Could you check a few things on this model? Use its own coordinates, in mm. Coordinates: 2 decimals unless noted, no trailing zeros. Order: outer loops, then holes, each group sorted by start corner. A loop starts at its lowest first (then second) coordinate and runs counter-clockwise, first axis right, second up. Notation, with made-up numbers: (66, -14.5) - (86, -14.5) arc R17 cw to (86, 2.5) - close; hole circle Ø6 at (14, 63.5). An arc over 180 degrees is marked (long way). Answer as a JSON object with one key per item and string values. Group by question number.
(1) Imagine slicing it at B-B, the plane y = 26.5. Write out the boundary of the cut face in (x, z).
(2) Will these pins go through, and if not, where does the flat tip stop? P1, Ø1.5, axis at x = 1.5, y = -37, coming from the -Z side; P2, Ø0.9, axis at x = 1.5, z = 45.5, coming from the -Y side; P3, Ø1.5, axis at x = 0.5, y = 30, coming from the +Z side.
(3) Please list where these lines run through material, in increasing order: probe 1 along Y at (x, z) = (1.95, -110); probe 2 along Z at (x, y) = (2.3, -20); probe 3 along Y at (x, z) = (2, -118.5).
(4) Imagine slicing it at A-A, the plane z = -119. Write out the boundary of the cut face in (x, y), and give its area (3 significant figures).
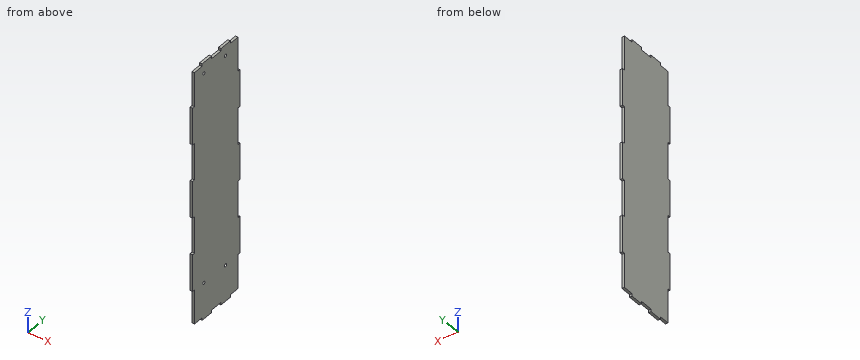
from build123d import *

# Parameters (mm, degrees)
BOSS_EXTRU_3_DEPTH                  = 3
DIAM_TRE_DU_PER_AGE_3_5_3_5_1_D     = 3.5
DIAM_TRE_DU_PER_AGE_3_5_3_5_1_DEPTH = 2
DIAM_TRE_DU_PER_AGE_3_5_3_5_1_TIP   = 1.051506083


with BuildPart() as part:
    # Esquisse3 → Boss.-Extru.3 (new body)
    with BuildSketch(Plane(origin=(0, 0, 0), x_dir=(0, 0, -1), z_dir=(1, 0, 0))):
        Polygon((109.285714286, 38), (65.571428571, 38), (65.571428571, 35), (21.857142857, 35), (21.857142857, 38), (-21.857142857, 38), (-21.857142857, 35), (-65.571428571, 35), (-65.571428571, 38), (-109.285714286, 38), (-109.285714286, 35), (-150, 35), (-150, 22.8), (-153, 22.8), (-153, 7.6), (-150, 7.6), (-150, -7.6), (-153, -7.6), (-153, -22.8), (-150, -22.8), (-150, -35), (-109.285714286, -35), (-109.285714286, -38), (-65.571428571, -38), (-65.571428571, -35), (-21.857142857, -35), (-21.857142857, -38), (21.857142857, -38), (21.857142857, -35), (65.571428571, -35), (65.571428571, -38), (109.285714286, -38), (109.285714286, -35), (150, -35), (150, -22.8), (153, -22.8), (153, -7.6), (150, -7.6), (150, 7.6), (153, 7.6), (153, 22.8), (150, 22.8), (150, 35), (109.285714286, 35), align=None)
    extrude(amount=BOSS_EXTRU_3_DEPTH)

    # Diamètre du perçage Ø3.5 (3.5)1
    with Locations(Plane(origin=(3, 0, 0), x_dir=(0, 0, -1), z_dir=(1, 0, 0))):
        with Locations((110, 15), (110, -20), (-140, 15), (-140, -20)):
            Hole(DIAM_TRE_DU_PER_AGE_3_5_3_5_1_D / 2, depth=DIAM_TRE_DU_PER_AGE_3_5_3_5_1_DEPTH)
            with Locations((0, 0, -(DIAM_TRE_DU_PER_AGE_3_5_3_5_1_DEPTH + DIAM_TRE_DU_PER_AGE_3_5_3_5_1_TIP / 2))):  # 118° drill point
                Cone(0, DIAM_TRE_DU_PER_AGE_3_5_3_5_1_D / 2, DIAM_TRE_DU_PER_AGE_3_5_3_5_1_TIP, mode=Mode.SUBTRACT)


solid = part.part
Result set:
{
 "1": {"outline": "(0, -150) - (3, -150) - (3, 150) - (0, 150) - close"},
 "2": {"P1": "stops at z = -109.29", "P2": "stops at y = -35", "P3": "stops at z = 150"},
 "3": {"probe 1": "y = -35 to -21.75, -18.25 to 13.25, 16.75 to 35", "probe 2": "z = -153 to -111.75, -108.25 to 138.25, 141.75 to 153", "probe 3": "y = -35 to 35"},
 "4": {"outline": "(0, -35) - (3, -35) - (3, 35) - (0, 35) - close", "area": "210 mm^2"}
}
